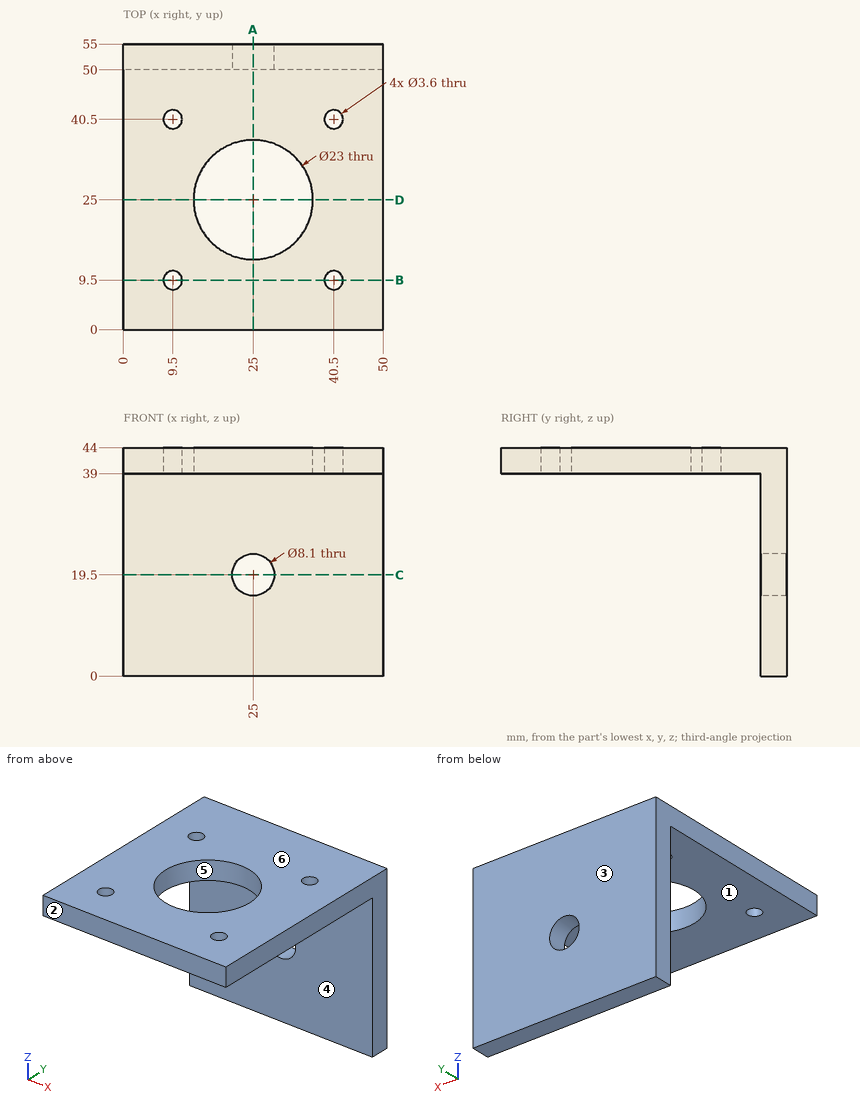
Answer from the drawing. Dimensions are ordinates in mm from the lowest x, y and z of the part. A direction names the side the tool comes from. Coordinates: 2 decimals unless noted, no trailing zeros. Order: outer loops, then holes, each group sorted by start corner. A loop starts at its lowest first (then second) coordinate and runs counter-clockwise, first axis right, second up. Notation, with made-up numbers: (31, -32) - (56, -32) arc R7 ccw to (56, -20) - close; hole circle Ø10 at (-27, 0.25). An arc over 180 degrees is marked (long way). Put each result on its own line as item: value. Start each with the question number.
1) Find section A-A (x = 25). Give the vertices of the cut face in (y, z).
2) For the marked faces 1 and 2, determine the directions among +Z, -Z, +X, -X, +Y, -Y from which every point of the face is accessible in a straight line to the end or side of a thin tool.
3) Find section C-C (z = 19.5). Give the vertices of the cut face in (x, y), plus the area to 4 significant figures.
4) For a pull along Y with two mould halves and no side action, classify the marked faces 3, 4, 5 and 6 as released by +Y, released by -Y, zero draft, split by the parting line, or undercut.
5) Flat-ended cylindrical pins translate along their axes: pin 1 (3 mm diameter, centred on x = 40.5, y = 9.5, fed in from -Z); pin 2 (19.5 mm diameter, centred on x = 22, z = 27.5, fed in from -Y); pin 3 (1.5 mm diameter, centred on x = 13.5, y = 22, fed in from -Z). Find the tip coordinate at first contact, or state that the pin passes through.
6) Find section B-B (y = 9.5). Give the vertices of the cut face in (x, z).
7) Find section D-D (y = 25). Give the vertices of the cut face in (x, z), plus the area to 3 significant figures.
8) Find the intervals of material crossed by line 1 (Y direction, x = 40.5, z = 42.5); line 2 (Y direction, x = 40, z = 40); line 3 (Z direction, x = 8, y = 20), in increasing order. Write a range as from..to.
Results list:
1. outline: (0, 39) - (13.5, 39) - (13.5, 44) - (0, 44) - close; (36.5, 39) - (50, 39) - (50, 23.55) - (55, 23.55) - (55, 44) - (36.5, 44) - close; (50, 0) - (55, 0) - (55, 15.45) - (50, 15.45) - close
2. face 1: -Z, +X, -X, -Y
2. face 2: +Z, -Z, +X, -X, -Y
3. outline: (0, 50) - (20.95, 50) - (20.95, 55) - (0, 55) - close; (29.05, 50) - (50, 50) - (50, 55) - (29.05, 55) - close
3. area: 209.5 mm^2
4. face 3: released by +Y
4. face 4: released by -Y
4. face 5: undercut
4. face 6: zero draft
5. pin 1: passes through
5. pin 2: stops at y = 50
5. pin 3: stops at z = 39
6. outline: (0, 39) - (7.7, 39) - (7.7, 44) - (0, 44) - close; (11.3, 39) - (38.7, 39) - (38.7, 44) - (11.3, 44) - close; (42.3, 39) - (50, 39) - (50, 44) - (42.3, 44) - close
7. outline: (0, 39) - (13.5, 39) - (13.5, 44) - (0, 44) - close; (36.5, 39) - (50, 39) - (50, 44) - (36.5, 44) - close
7. area: 135 mm^2
8. line 1: y = 0..7.7, 11.3..38.7, 42.3..55
8. line 2: y = 0..7.77, 11.23..38.77, 42.23..55
8. line 3: z = 39..44
